Read the model definition and answer for the solid it produces. Units are mm, in the model's axes. A direction names the side the tool comes from. Coordinates: 2 decimals unless noted, no trailing zeros. Order: outer loops, then holes, each group sorted by start corner. A loop starts at its lowest first (then second) coordinate and runs counter-clockwise, first axis right, second up. Notation, with made-up numbers: M -2.5,32 L 7.5,32 A32 ccw 7.5,66 Z; hole C 82,39 d4. An arc over 180 degrees is marked long. Write each question's results on one line, items separated by ' | '.
```python
from build123d import *

# Parameters (mm, degrees)
F0_R          = 49.1744
F1_DEPTH      = 57.15
F4_W          = 6.35
F4_H          = 57.15
F5_DEPTH      = 127
F5_DEPTH_BACK = 17.018
F6_R          = 3.175
F7_DEPTH      = 57.15
F8_W          = 25.4
F8_H          = 25.4
F9_DEPTH      = 50.8


with BuildPart() as f1:
    # F0 (on Top) → F1 (new body)
    with BuildSketch(Plane.XY):
        Circle(F0_R)
    extrude(amount=F1_DEPTH)

    # F2 (on Front) → F3 (revolve, cut)
    with BuildSketch(Plane.XZ):
        with BuildLine():
            Line((0, 57.15), (-48.26, 57.15))
            ThreePointArc((-48.26, 57.15), (-34.1249732601, 23.0250267399), (0, 8.89))
            Line((0, 8.89), (0, 57.15))
        make_face()
    revolve(axis=Axis((0, 0, 33.02), (0, 0, -1)), mode=Mode.SUBTRACT)

    # F4 (on Front) → F5 (cut, two sides)
    with BuildSketch(Plane.XZ) as f5_sk:
        with Locations((0, 28.575)):
            Rectangle(F4_W, F4_H)
    extrude(amount=-F5_DEPTH, mode=Mode.SUBTRACT)
    extrude(f5_sk.sketch, amount=F5_DEPTH_BACK, mode=Mode.SUBTRACT)

    # F6 (on Top) → F7 (join)
    with BuildSketch(Plane.XY):
        with BuildLine():
            ThreePointArc((24.742076835, -42.4964851399), (0, -49.1744), (-24.742076835, -42.4964851399))
            Line((-24.742076835, -42.4964851399), (-24.742076835, -80.5964851399))
            Line((-24.742076835, -80.5964851399), (24.742076835, -80.5964851399))
            Line((24.742076835, -80.5964851399), (24.742076835, -42.4964851399))
        make_face()
        with Locations((0, -74.2464851399)):
            Circle(F6_R, mode=Mode.SUBTRACT)
    extrude(amount=F7_DEPTH)

    # F8 (on face) → F9 (cut)
    with BuildSketch(Plane(origin=(-24.742076835, 0, 0), x_dir=(0, -1, 0), z_dir=(-1, 0, 0))):
        with Locations((67.8964851399, 28.575)):
            Rectangle(F8_W, F8_H)
    extrude(amount=-F9_DEPTH, mode=Mode.SUBTRACT)


solid = f1.part
```
(1) The part is cut by section A-A, the plane y = -58. Write down the section's boundary in (x, z) (3 decimals), then the cut area to 3 significant figures.
Conclusion:
outline: M -24.742,0 L 24.742,0 L 24.742,15.875 L -24.742,15.875 Z; M -24.742,41.275 L 24.742,41.275 L 24.742,57.15 L -24.742,57.15 Z | area: 1,570 mm²
(2) Straight lines are drawn through the part: line 1 (Y direction, x = 0, z = 7.5); line 2 (Z direction, x = -24.5, y = -67.5) (3 decimals); line 3 (Y direction, x = 0, z = 50). For each, find the intervals that lie inside material, in ascending order.
Conclusion:
line 1: -80.6 to -77.42, -71.07 to -17.02 | line 2: 0 to 15.875, 41.275 to 57.15 | line 3: -80.6 to -77.42, -71.07 to -47.73
(3) Given pin 1 (8 mm diameter, centred on y = -20, z = 36, fed in from -X); pin 2 (7.5 mm diameter, centred on x = 9, z = 25.5, fed in from -Y); pin 3 (1 mm diameter, centred on x = -18, z = 11.5, fed in from +Y), each flat-ended and moving along its own axis, determine where each tip first touches the part or whether it passes through.
Conclusion:
pin 1: x = -46.5 | pin 2: y = -55.2 | pin 3: y = 45.96
(4) The part is cut by section C-C, the plane y = 2. Write down the section's boundary in (x, z) (3 decimals).
Conclusion:
outline: M -49.134,0 L -3.175,0 L -3.175,9.036 A48.219 cw -48.219,57.15 L -49.134,57.15 Z; M 3.175,0 L 49.134,0 L 49.134,57.15 L 48.219,57.15 A48.219 cw 3.175,9.036 Z
(5) The mould has two halves that part along X. Classify faces 1 (the cylindrical face through (-0.41, -71.1, 49.1)), 2 (the cylindrical face through (48.058, 10.418, 28.175)), 3 (the flat face through (0, -55.196, 28)): pulls with the +X half, pulls with the -X half, needs draft (parallel to the pull), parting line crosses it, or undercut.
Conclusion:
face 1: undercut | face 2: pulls with the +X half | face 3: needs draft
(6) For faces 4 (the flat face through (0, -68, 15.875)), 5 (the cylindrical face through (-47.656, 12.126, 28.175)), 6 (the flat face through (-24.742, -53, 28)), 7 (the flat face through (3.175, 26, 14)), 8 (the flat face through (24.742, -53, 28)), determine the directions among +Z, -Z, +X, -X, +Y, -Y from which every point of the face is accessible in a straight line to the end or side of a thin tool.
Conclusion:
face 4: +X, -X, -Y | face 5: +Z, -Z, -X | face 6: +Z, -Z, -X, -Y | face 7: +Z, -Z, +Y | face 8: +Z, -Z, +X, -Y
(7) The part is cut by section B-B, the plane x = 0. Write down the section's boundary in (y, z) (3 decimals).
Conclusion:
outline: M -80.596,0 L -77.421,0 L -77.421,15.875 L -80.596,15.875 Z; M -80.596,41.275 L -77.421,41.275 L -77.421,57.15 L -80.596,57.15 Z; M -71.071,0 L -17.018,0 L -17.018,11.99 A48.26 cw -48.26,57.15 L -71.071,57.15 L -71.071,41.275 L -55.196,41.275 L -55.196,15.875 L -71.071,15.875 Z
(8) The part is cut by section D-D, the plane x = 18.5. Write down the section's boundary in (y, z) (3 decimals), then the cut area to 3 significant figures.
Conclusion:
outline: M -80.596,0 L 45.562,0 L 45.562,57.15 L 44.573,57.15 A44.573 cw -44.573,57.15 L -80.596,57.15 L -80.596,41.275 L -55.196,41.275 L -55.196,15.875 L -80.596,15.875 Z | area: 3,440 mm²
